from build123d import *

# Parameters (mm, degrees)
F0_W      = 33.4
F0_H      = 23
F1_DEPTH  = 8
F0_W_2    = 17.8890476892
F0_H_2    = 16.5
F2_DEPTH  = 4.5
F3_DEPTH  = 1
F4_DEPTH  = 1
F5_DEPTH  = 1
F6_DEPTH  = 1
F7_DEPTH  = 2
F8_W      = 13.3992488682
F8_H      = 12.2999999374
F9_DEPTH  = 3.4
F11_W     = 28.4
F11_H     = 5
F12_DEPTH = 0.75
F13_W     = 28.4
F13_H     = 5
F14_DEPTH = 0.75
F15_W     = 18
F15_H     = 5
F16_DEPTH = 1.75
F10_W     = 16.5
F10_H     = 8
F17_DEPTH = 2.5
F18_R     = 0.99999


# Not quite as in the source:
# - a fillet or chamfer is up to 0.001 mm smaller than in the source, because OpenCascade refuses the exact size
# - a feature names something its author has since deleted; it is built from what else it names


with BuildPart() as f1:
    # F0 (on Top) → F1 (new body)
    with BuildSketch(Plane.XY):
        with Locations((-3.299, -0.375)):
            Rectangle(F0_W, F0_H)
        Polygon((1.3400476892, 7.875), (9.951, 7.875), (9.951, -8.625), (1.3400476892, -8.625), (-16.549, -8.625), (-16.549, 7.875), align=None, mode=Mode.SUBTRACT)
    extrude(amount=F1_DEPTH)

    # F0 (on Top) → F2 (join)
    with BuildSketch(Plane.XY):
        with Locations((-7.6044761554, -0.375)):
            Rectangle(F0_W_2, F0_H_2)
    extrude(amount=F2_DEPTH)

    # F3 (cut): a face of the model
    f3_faces = [f1.faces().sort_by_distance(p)[0] for p in [
        (-3.299, -11.875, 4),
    ]]
    extrude(f3_faces, amount=-F3_DEPTH, mode=Mode.SUBTRACT)

    # F4 (cut): a face of the model
    f4_faces = [f1.faces().sort_by_distance(p)[0] for p in [
        (13.401, 0.125, 4),
    ]]
    extrude(f4_faces, amount=-F4_DEPTH, mode=Mode.SUBTRACT)

    # F5 (cut): a face of the model
    f5_faces = [f1.faces().sort_by_distance(p)[0] for p in [
        (-3.799, 11.125, 4),
    ]]
    extrude(f5_faces, amount=-F5_DEPTH, mode=Mode.SUBTRACT)

    # F6 (cut): a face of the model
    f6_faces = [f1.faces().sort_by_distance(p)[0] for p in [
        (-19.999, -0.375, 4),
    ]]
    extrude(f6_faces, amount=-F6_DEPTH, mode=Mode.SUBTRACT)

    # F0 (on Top) → F7 (cut)
    with BuildSketch(Plane.XY):
        with Locations((-7.6044761554, -0.375)):
            Rectangle(F0_W_2, F0_H_2)
    extrude(amount=F7_DEPTH, mode=Mode.SUBTRACT)

    # F8 (on face) → F9 (cut)
    with BuildSketch(Plane(origin=(0, 0, 2), x_dir=(1, 0, 0), z_dir=(0, 0, -1))):
        with Locations((-7.7493755346, 0.375)):
            Rectangle(F8_W, F8_H)
    extrude(amount=-F9_DEPTH, mode=Mode.SUBTRACT)

    # F11 (on face) → F12 (cut)
    with BuildSketch(Plane.XZ.offset(10.875)):
        with Locations((-3.299, 4)):
            Rectangle(F11_W, F11_H)
    extrude(amount=-F12_DEPTH, mode=Mode.SUBTRACT)

    # F13 (on face) → F14 (cut)
    with BuildSketch(Plane(origin=(0, 10.125, 0), x_dir=(-1, 0, 0), z_dir=(0, 1, 0))):
        with Locations((3.299, 4)):
            Rectangle(F13_W, F13_H)
    extrude(amount=-F14_DEPTH, mode=Mode.SUBTRACT)

    # F15 (on face) → F16 (cut)
    with BuildSketch(Plane(origin=(-18.999, 0, 0), x_dir=(0, -1, 0), z_dir=(-1, 0, 0))):
        with Locations((0.375, 4)):
            Rectangle(F15_W, F15_H)
    extrude(amount=-F16_DEPTH, mode=Mode.SUBTRACT)

    # F10 (on face) → F17 (cut)
    with BuildSketch(Plane.YZ.offset(12.401)):
        with Locations((-0.375, 4)):
            Rectangle(F10_W, F10_H)
    extrude(amount=-F17_DEPTH, mode=Mode.SUBTRACT)

    # F18 (radius 1 in the source; OpenCascade refuses exactly that, so slightly less here)
    f18_edges = [f1.edges().sort_by_distance(p)[0] for p in [
        (-3.299, 10.125, 8),
        (-2.074, 7.875, 8),
        (-18.999, -0.375, 8),
        (-16.549, -0.375, 8),
        (-2.074, -8.625, 8),
        (-3.299, -10.875, 8),
        (12.401, -9.75, 8),
        (12.401, 9, 8),
        (12.401, 9, 0),
        (12.401, -9.75, 0),
        (-3.299, 10.125, 0),
        (-3.299, -10.875, 0),
        (-18.999, -0.375, 0),
        (-2.074, -8.625, 0),
        (-16.549, -0.375, 0),
        (-2.074, 7.875, 0),
        (12.401, -10.875, 4),
        (12.401, -8.625, 4),
        (12.401, 7.875, 4),
        (12.401, 10.125, 4),
        (-18.999, -10.875, 4),
        (-18.999, 10.125, 4),
        (-14.449, -0.375, 4.5),
        (-1.049751, -0.375, 4.5),
        (-7.604476, 7.875, 2),
        (-16.549, -0.375, 2),
        (-7.604476, -8.625, 2),
        (-1.049751, -0.375, 2),
        (-14.449, -0.375, 2),
        (-16.549, -0.375, 4.5),
        (1.340048, -0.375, 4.5),
        (1.340048, -0.375, 2),
        (1.340048, 7.875, 3.25),
        (-7.604476, 7.875, 4.5),
        (-7.604476, -8.625, 4.5),
        (-7.749376, -6.525, 4.5),
        (-7.749376, 5.775, 4.5),
        (1.340048, -8.625, 3.25),
    ]]
    fillet(f18_edges, radius=F18_R)


solid = f1.part
Read the model definition and answer for the solid it produces. Units are mm, in the model's axes. A direction names the side the tool comes from. Round coordinates to 2 decimals unless told otherwise and drop trailing zeros. Order: outer loops, then holes, each group sorted by start corner. A loop starts at its lowest first (then second) coordinate and runs counter-clockwise, first axis right, second up. Notation, with made-up numbers: (38, 55) - (72, 55) arc R20 cw to (72, 77) - close; hole circle Ø6 at (14.5, -16.5). An arc over 180 degrees is marked (long way). Use one line per item in the form item = value. Start each with the question number.
(1) Find the intervals of material crossed by line 1 along Y through (x, z) = (1.5, 1.25) (3 decimals); line 2 along X through (y, z) = (-4, 3.5); line 3 along Y through (x, z) = (-4.5, 2.5) (3 decimals), in increasing order. Write a range as from..to.
(2) For faces 5 (the face through (-2.87, -8.91, 0.3)), 6 (the face through (-14.734, -0.275, 4.199)), 7 (the face through (-3.09, -10.59, 7.7)), 8 (the face through (-18, -9.375, 4)), 9 (the face through (1.055, -0.273, 4.199)), determine the directions among +Z, -Z, +X, -X, +Y, -Y from which every point of the face is accessible in a straight line to the end or side of a thin tool.
(3) Flat-ended cylindrical pins translate along their axes: pin 1 Ø2 at (y, z) = (0.5, 4) entering from +X; pin 2 Ø3 at (x, z) = (3, 3.5) entering from -Y (3 decimals); pin 3 Ø1 at (x, y) = (-6.5, -7.5) entering from +Z. Find the tip coordinate at first contact, or state that the pin passes through.
(4) The part is cut by section C-C (z = 0.5). Give the vertices of the cut face in (x, y) (3 decimals).
(5) The part is cut by section B-B (x = 4.5). Give the vertices of the cut face in (y, z) (3 decimals).
(6) Determine the mould class of faces 1 (the face through (12.12, -10.57, 4.04)), 2 (the face through (1.055, -0.273, 2.301)), 3 (the face through (-3.09, 9.84, 7.7)), 4 (the face through (-0.749, -0.461, 2.285)) for opening direction Y: +Y half, -Y half, draft (parallel to the pull), parting line (faces both ways), or undercut.
Checked values:
q1.line_1 = -10.875..-8.625, 7.875..10.125
q1.line_2 = -17.25..-14.45, -1.05..1.34
q1.line_3 = -10.125..-6.525, 5.775..9.375
q2.face_5 = -Z, +X
q2.face_6 = +Z
q2.face_7 = +Z, +X, -X, -Y
q2.face_8 = -X
q2.face_9 = +Z, +X
q3.pin_1 = 1.34
q3.pin_2 = -10.125
q3.pin_3 = 4.57
q4.outline = (-18.865, -9.875) arc R0.866 ccw to (-17.999, -10.741) - (11.401, -10.741) arc R0.866 ccw to (12.267, -9.875) - (12.267, -9.625) arc R0.866 ccw to (11.401, -8.759) - (-16.683, -8.759) - (-16.683, 8.009) - (11.401, 8.009) arc R0.866 ccw to (12.267, 8.875) - (12.267, 9.125) arc R0.866 ccw to (11.401, 9.991) - (-17.999, 9.991) arc R0.866 ccw to (-18.865, 9.125) - close
q5.outline = (-10.875, 1) arc R1 ccw to (-9.875, 0) - (-9.625, 0) arc R1 ccw to (-8.625, 1) - (-8.625, 7) arc R1 ccw to (-9.625, 8) - (-9.875, 8) arc R1 ccw to (-10.875, 7) - (-10.875, 6.5) - (-10.125, 6.5) - (-10.125, 1.5) - (-10.875, 1.5) - close; (7.875, 1) arc R1 ccw to (8.875, 0) - (9.125, 0) arc R1 ccw to (10.125, 1) - (10.125, 1.5) - (9.375, 1.5) - (9.375, 6.5) - (10.125, 6.5) - (10.125, 7) arc R1 ccw to (9.125, 8) - (8.875, 8) arc R1 ccw to (7.875, 7) - close
q6.face_1 = -Y half
q6.face_2 = undercut
q6.face_3 = +Y half
q6.face_4 = undercut
